Part model, mm, in its own coordinate system. A direction names the side the tool comes from. Give positions to 0.01 mm unless a question says otherwise; leave off trailing zeros. Order: outer loops, then holes, each group sorted by start corner. A loop starts at its lowest first (then second) coordinate and runs counter-clockwise, first axis right, second up. Notation, with made-up numbers: (23, -23) - (70, -23) arc R29 ccw to (70, -2) - close; hole circle Ø2 at (26, -18). An arc over 180 degrees is marked (long way). Use one line per item in the form item = value. Start each with the question number.
1. Tool access for faces 1 (the face through (0, -9, -14.288)), 2 (the face through (0, -4, -17.462)), 3 (the face through (0, 9, -17.462)), 4 (the face through (0, -1.588, 11)): list every direction of +Z, -Z, +X, -X, +Y, -Y with a clear straight run to the whole face (end or side of a thin tool).
2. Band-saw the part on D-D, the plane x = -4. List the corners of the cut face in (y, z).
3. Band-saw the part on B-B, the plane y = 4.25. List the corners of the cut face in (x, z), plus the area to 3 significant figures.
4. Pin check, flat tips, straight feed: P1, Ø1, axis at x = 3.5, z = -4.5, coming from the -Y side; P2, Ø6, axis at y = -0.5, z = -21.5, coming from the -X side; P3, Ø0.5, axis at x = 2.5, y = -9, coming from the +Z side; P4, Ø1.3, axis at x = -2, y = 9, coming from the -Z side. Stop position of each tip, or through.
5. Drill centre lines: line 1 (Z direction, x = -3.25, y = 0); line 2 (Y direction, x = 0.75, z = -23); line 3 (Y direction, x = 4.25, z = -3.5). Where is each one in solid material? Low to high.
6. Band-saw the part on A-A, the plane x = 2.25. List the corners of the cut face in (y, z) (1 decimal), plus the area to 3 significant figures.
7. Band-saw the part on C-C, the plane z = -26. List the corners of the cut face in (x, y), plus the area to 3 significant figures.
Autodesk Inventor part; units mm, degrees
ref_plane "YZ Plane" through (0, 0, 0) normal (1, 0, 0) x (0, 1, 0)
ref_plane "XZ Plane" through (0, 0, 0) normal (0, 1, 0) x (-1, 0, 0)
ref_plane "XY Plane" through (0, 0, 0) normal (0, 0, 1) x (1, 0, 0)
sketch "Sketch1" plane through (0, 0, 0) normal (1, 0, 0) x (0, 1, 0)
  line L0 (-9.525, 36.5125) -> (9.525, 36.5125)
  line L1 (9.525, 36.5125) -> (9.525, -36.5125)
  line L2 (9.525, -36.5125) -> (-9.525, -36.5125)
  line L3 (-9.525, -36.5125) -> (-9.525, 36.5125)
  line L4 (-9.525, 36.5125) -> (9.525, -36.5125) construction
  line L5 (9.525, 36.5125) -> (-9.525, -36.5125) construction
  point P0 (0, 0)
  dimension "d0" = 19.05
  dimension "d1" = 73.025
extrude "Extrusion1" add sketch "Sketch1" along normal mid plane 9.525
sketch "Sketch2" plane through (4.7625, 0, 0) normal (1, 0, 0) x (0, 0, -1)
  line L0 (-36.5125, 9.525) -> (-36.5125, -9.525)
  line L1 (-36.5125, 9.525) -> (14.2875, 9.525)
  line L2 (14.2875, 9.525) -> (14.2875, -1.5875)
  line L3 (14.2875, -1.5875) -> (-36.5125, -1.5875)
  line L4 (-36.5125, -1.5875) -> (-36.5125, 9.525)
  line L5 (-36.5125, -9.525) -> (36.5125, -9.525)
  point P0 (0, 0)
  dimension "d4" = 50.8
  dimension "d6" = 7.9375
extrude "Extrusion2" cut sketch "Sketch2" against normal blind 9.525
sketch "Sketch3" plane through (4.7625, 0, 0) normal (1, 0, 0) x (0, 0, -1)
  line L0 (36.5125, -9.525) -> (-36.5125, -9.525)
  line L1 (36.5125, -9.525) -> (17.4625, -9.525)
  line L2 (17.4625, -9.525) -> (17.4625, 1.5875)
  line L3 (17.4625, 1.5875) -> (36.5125, 1.5875)
  line L4 (36.5125, 1.5875) -> (36.5125, -9.525)
  line L5 (14.2875, 9.525) -> (14.2875, -1.5875)
  line L6 (36.5125, 9.525) -> (14.2875, 9.525)
  point P0 (0, 0)
  dimension "d9" = 3.175
  dimension "d10" = 7.9375
extrude "Extrusion3" cut sketch "Sketch3" against normal blind 9.525
sketch "Sketch4" plane through (4.7625, 0, 0) normal (1, 0, 0) x (0, 0, -1)
  line L0 (-36.5125, -1.5875) -> (-36.5125, -9.525)
  line L1 (-36.5125, -9.525) -> (14.2875, -9.525)
  line L2 (14.2875, -9.525) -> (14.2875, -7.9375)
  line L3 (14.2875, -7.9375) -> (-36.5125, -7.9375)
  line L4 (-36.5125, -7.9375) -> (-36.5125, -9.525)
  point P0 (0, 0)
  dimension "d13" = 50.8
  dimension "d14" = 1.5875
extrude "Extrusion4" cut sketch "Sketch4" against normal blind 9.525
sketch "Sketch5" plane through (4.7625, 0, 0) normal (1, 0, 0) x (0, 0, -1)
  line L0 (36.5125, 9.525) -> (36.5125, 1.5875)
  line L1 (36.5125, 9.525) -> (17.4625, 9.525)
  line L2 (17.4625, 9.525) -> (17.4625, 7.9375)
  line L3 (17.4625, 7.9375) -> (36.5125, 7.9375)
  line L4 (36.5125, 7.9375) -> (36.5125, 9.525)
  point P0 (0, 0)
  dimension "d17" = 19.05
  dimension "d18" = 1.5875
extrude "Extrusion5" cut sketch "Sketch5" against normal blind 9.525
fillet "Fillet1" radius 1.5875 4 edges at (4.7625, 9.525, -15.875) (-4.7625, 9.525, -15.875) (4.7625, -9.525, -15.875) (-4.7625, -9.525, -15.875)
properties part number "CrankShaft Mill"
From the geometry:
q1.face_1 = +Z, +X, -X, -Y
q1.face_2 = -Z, +X, -X, -Y
q1.face_3 = -Z, +X, -X, +Y
q1.face_4 = +Z, +X, -X, +Y
q2.outline = (-9.29, -17.46) - (1.59, -17.46) - (1.59, -36.51) - (7.94, -36.51) - (7.94, -17.46) - (9.29, -17.46) - (9.29, -14.29) - (-1.59, -14.29) - (-1.59, 36.51) - (-7.94, 36.51) - (-7.94, -14.29) - (-9.29, -14.29) - close
q3.outline = (-4.76, -36.51) - (4.76, -36.51) - (4.76, -14.29) - (-4.76, -14.29) - close
q3.area = 212 mm²
q4.P1 = -7.94
q4.P2 = -4.76
q4.P3 = -14.29
q4.P4 = -17.46
q5.line_1 = -17.46 to -14.29
q5.line_2 = 1.59 to 7.94
q5.line_3 = -7.94 to -1.59
q6.outline = (-9.5, -17.5) - (1.6, -17.5) - (1.6, -36.5) - (7.9, -36.5) - (7.9, -17.5) - (9.5, -17.5) - (9.5, -14.3) - (-1.6, -14.3) - (-1.6, 36.5) - (-7.9, 36.5) - (-7.9, -14.3) - (-9.5, -14.3) - close
q6.area = 504 mm²
q7.outline = (-4.76, 1.59) - (4.76, 1.59) - (4.76, 7.94) - (-4.76, 7.94) - close
q7.area = 60.5 mm²
